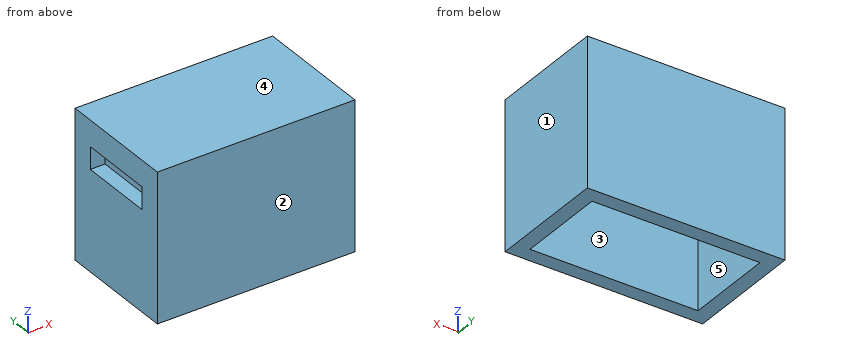
from build123d import *

# Parameters (mm, degrees)
SKETCH1_W           = 22.7
SKETCH1_H           = 12.2
BOSS_EXTRUDE1_DEPTH = 3.5
SKETCH2_W           = 26.7
SKETCH2_H           = 16.2
SKETCH2_W_2         = 22.7
SKETCH2_H_2         = 12.2
BOSS_EXTRUDE2_DEPTH = 20
SKETCH3_W           = 3
SKETCH3_H           = 10.2
CUT_EXTRUDE1_DEPTH  = 2


with BuildPart() as part:
    # Sketch1 → Boss-Extrude1 (new body)
    with BuildSketch(Plane.XY):
        Rectangle(SKETCH1_W, SKETCH1_H)
    extrude(amount=BOSS_EXTRUDE1_DEPTH)

    # Sketch2 → Boss-Extrude2 (add)
    with BuildSketch(Plane.XY.offset(3.5)):
        Rectangle(SKETCH2_W, SKETCH2_H)
        Rectangle(SKETCH2_W_2, SKETCH2_H_2, mode=Mode.SUBTRACT)
    extrude(amount=-BOSS_EXTRUDE2_DEPTH)

    # Sketch3 → Cut-Extrude1 (cut)
    with BuildSketch(Plane.ZY.offset(13.35)):
        with Locations((-1.5, 0)):
            Rectangle(SKETCH3_W, SKETCH3_H)
    extrude(amount=-CUT_EXTRUDE1_DEPTH, mode=Mode.SUBTRACT)


solid = part.part
Source: CAD feature listing. Evaluate the final solid. Frame: model axes, mm. Face numbers are marked on the shaded views. A direction names the side the tool comes from. Round coordinates to 2 decimals unless told otherwise and drop trailing zeros. Loops run counter-clockwise (first coordinate to the right, second up) from the corner with the lowest first, then second, coordinate; pieces in that order, holes last. Notation, with made-up numbers: M -15.75,46.25 L -7.75,46.25 A19 ccw -7.75,68.25 Z; hole C 65.5,-1 d9. An arc over 180 degrees is marked long. Return JSON: item names as keys, results as strings. Group by question number.
1. Mould query, pull axis X, two halves, no side actions, for the marked faces 1, 2 and 3. Classes: released by +X, released by -X, zero draft, split by the parting line, or undercut.
2. Section query B-B on z = -12.5. Output: boundary loops of the cut face in (x, y).
3. Material intervals for line 1 along X through (y, z) = (4.25, -9.25); line 2 along Y through (x, z) = (0.5, -12.75); line 3 along Z through (x, y) = (-1.75, 5), sorted ascending. Write a range as from..to.
4. Section query A-A on y = -4.5. Output: boundary loops of the cut face in (x, z), and give its area (3 significant figures).
5. Reachability of the marked faces 4 and 5 from +Z, -Z, +X, -X, +Y, -Y: full face, straight path, thin tool, end or side. Return the list, or none.
6. Pin query (flat end, axial travel): pin 1 (1 mm diameter, centred on x = 1.5, y = 2.5, fed in from -Z). Return the tip coordinate at first contact, or that it passes through.
7. Section query C-C on x = 8.75. Output: boundary loops of the cut face in (y, z), and give its area (3 significant figures).
Checks:
{
 "1": {"face 1": "released by +X", "face 2": "zero draft", "face 3": "undercut"},
 "2": {"outline": "M -13.35,-8.1 L 13.35,-8.1 L 13.35,8.1 L -13.35,8.1 Z; hole M -11.35,-6.1 L 11.35,-6.1 L 11.35,6.1 L -11.35,6.1 Z"},
 "3": {"line 1": "x = -13.35..-11.35, 11.35..13.35", "line 2": "y = -8.1..-6.1, 6.1..8.1", "line 3": "z = 0..3.5"},
 "4": {"outline": "M -13.35,-16.5 L -11.35,-16.5 L -11.35,-3 L -13.35,-3 Z; M -13.35,0 L 11.35,0 L 11.35,-16.5 L 13.35,-16.5 L 13.35,3.5 L -13.35,3.5 Z", "area": "153 mm²"},
 "5": {"face 4": "+Z, +X, -X, +Y, -Y", "face 5": "-Z"},
 "6": {"pin 1": "stops at z = 0"},
 "7": {"outline": "M -8.1,-16.5 L -6.1,-16.5 L -6.1,0 L 6.1,0 L 6.1,-16.5 L 8.1,-16.5 L 8.1,3.5 L -8.1,3.5 Z", "area": "123 mm²"}
}
